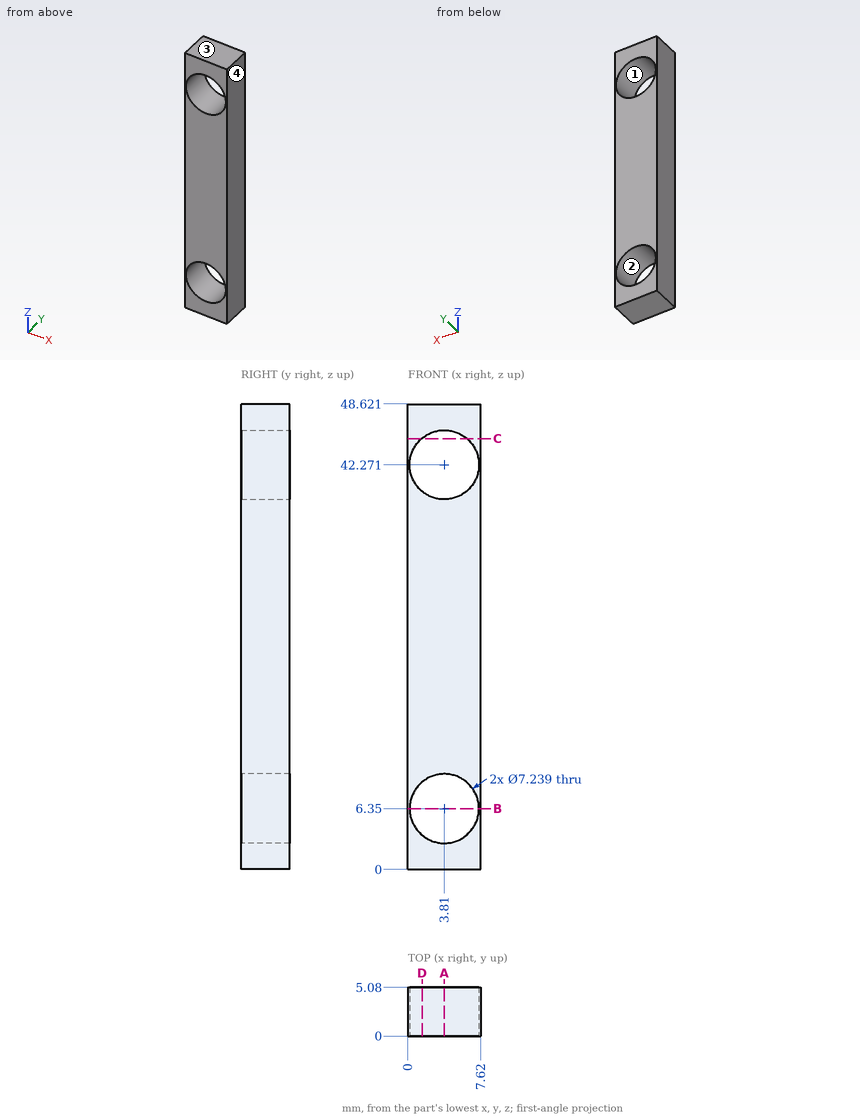
Geometry check sheet. Reference: drawing and pictorial views, mm from the part's lowest x, y, z. Give positions to 0.01 mm unless a question says otherwise; leave off trailing zeros. Order: outer loops, then holes, each group sorted by start corner. A loop starts at its lowest first (then second) coordinate and runs counter-clockwise, first axis right, second up. Notation, with made-up numbers: M 11.5,38.5 L 41.5,38.5 A21 cw 41.5,73.5 Z; hole C 8.25,52 d3. An arc over 180 degrees is marked long. Answer in a Markdown table with one row per item. Add a question column.
Q1. Sectioned sample at B-B, the plane z = 6.35. Record the boundary of the cut face in (x, y).
Q2. Sectioned sample at D-D, the plane x = 1.5. Record the boundary of the cut face in (y, z).
Q3. Thickness scan on L1, parallel to Z at x = 3.81, y = 2.45; L2, parallel to Z at x = 0.5, y = 4.75 (1 decimal); L3, parallel to X at y = 1.05, z = 9 (1 decimal). Record the ranges inside material, lowest first.
Q4. Sectioned sample at C-C, the plane z = 45. Record the boundary of the cut face in (x, y).
Q5. Sectioned sample at A-A, the plane x = 3.81. Record the boundary of the cut face in (y, z).
Q6. Release check for a two-part mould opening along Z. For the marked faces 1, 2, 3 and 4 record: released by +Z, released by -Z, zero draft, split by the parting line, or undercut.
Verdict:
| question | item | result |
|---|---|---|
| 1 | outline | M 0,0 L 0.19,0 L 0.19,5.08 L 0,5.08 Z; M 7.43,0 L 7.62,0 L 7.62,5.08 L 7.43,5.08 Z |
| 2 | outline | M 0,0 L 5.08,0 L 5.08,3.56 L 0,3.56 Z; M 0,9.14 L 5.08,9.14 L 5.08,39.48 L 0,39.48 Z; M 0,45.06 L 5.08,45.06 L 5.08,48.62 L 0,48.62 Z |
| 3 | L1 | 0 to 2.73, 9.97 to 38.65, 45.89 to 48.62 |
| 3 | L2 | 0 to 4.9, 7.8 to 40.8, 43.7 to 48.6 |
| 3 | L3 | 0 to 1.3, 6.3 to 7.6 |
| 4 | outline | M 0,0 L 1.43,0 L 1.43,5.08 L 0,5.08 Z; M 6.19,0 L 7.62,0 L 7.62,5.08 L 6.19,5.08 Z |
| 5 | outline | M 0,0 L 5.08,0 L 5.08,2.73 L 0,2.73 Z; M 0,9.97 L 5.08,9.97 L 5.08,38.65 L 0,38.65 Z; M 0,45.89 L 5.08,45.89 L 5.08,48.62 L 0,48.62 Z |
| 6 | face 1 | undercut |
| 6 | face 2 | undercut |
| 6 | face 3 | released by +Z |
| 6 | face 4 | zero draft |
